from build123d import *

# Parameters (mm, degrees)
SKETCH1_R           = 1.5
BOSS_EXTRUDE1_DEPTH = 1.2
SKETCH2_W           = 29.840930046
SKETCH2_H           = 54.765276652
BOSS_EXTRUDE2_DEPTH = 7
SKETCH3_W           = 33.788082064
SKETCH3_H           = 72.581353001
BOSS_EXTRUDE3_DEPTH = 5.5
SKETCH4_R           = 20
BOSS_EXTRUDE4_DEPTH = 16
SKETCH5_R           = 2.6
BOSS_EXTRUDE5_DEPTH = 6
BOSS_EXTRUDE6_DEPTH = 1.2
FILLET1_R           = 2.5


with BuildPart() as part:
    # Sketch1 → Boss-Extrude1 (new body)
    with BuildSketch(Plane(origin=(0, 0, 0), x_dir=(1, 0, 0), z_dir=(0, 1, 0))):
        with BuildLine():
            Line((2.5, 100), (97.5, 100))
            ThreePointArc((97.5, 100), (99.267766953, 99.267766953), (100, 97.5))
            Line((100, 97.5), (100, 2.5))
            ThreePointArc((100, 2.5), (99.267766953, 0.732233047), (97.5, 0))
            Line((97.5, 0), (2.5, 0))
            ThreePointArc((2.5, 0), (0.732233047, 0.732233047), (0, 2.5))
            Line((0, 2.5), (0, 97.5))
            ThreePointArc((0, 97.5), (0.732233047, 99.267766953), (2.5, 100))
        make_face()
        with Locations((5, 96.3)):
            Circle(SKETCH1_R, mode=Mode.SUBTRACT)
        with Locations((94.6, 95.1)):
            Circle(SKETCH1_R, mode=Mode.SUBTRACT)
        with Locations((5, 3.7)):
            Circle(SKETCH1_R, mode=Mode.SUBTRACT)
        with Locations((94.6, 4.4)):
            Circle(SKETCH1_R, mode=Mode.SUBTRACT)
    extrude(amount=BOSS_EXTRUDE1_DEPTH)

    # Sketch2 → Boss-Extrude2 (add)
    with BuildSketch(Plane.XZ):
        with Locations((36.983095354, -49.21487939)):
            Rectangle(SKETCH2_W, SKETCH2_H)
    extrude(amount=BOSS_EXTRUDE2_DEPTH)

    # Sketch3 → Boss-Extrude3 (add)
    with BuildSketch(Plane.XZ):
        with Locations((79.907693041, -55.955425872)):
            Rectangle(SKETCH3_W, SKETCH3_H)
    extrude(amount=BOSS_EXTRUDE3_DEPTH)

    # Sketch4 → Boss-Extrude4 (add)
    with BuildSketch(Plane(origin=(0, 1.2, 0), x_dir=(1, 0, 0), z_dir=(0, 1, 0))):
        with BuildLine():
            Line((23, -1), (23, 72))
            ThreePointArc((23, 72), (58.049844719, 97.772077914), (72.2, 56.63250183))
            ThreePointArc((72.2, 56.63250183), (69.818614724, 51.754066196), (69, 46.38750305))
            Line((69, 46.38750305), (69, -1))
            Line((69, -1), (23, -1))
        make_face()
        with Locations((50, 72)):
            Circle(SKETCH4_R, mode=Mode.SUBTRACT)
    extrude(amount=BOSS_EXTRUDE4_DEPTH)

    # Sketch5 → Boss-Extrude5 (add)
    with BuildSketch(Plane(origin=(0, 1.2, 0), x_dir=(1, 0, 0), z_dir=(0, 1, 0))):
        with Locations((87.841987056, 95.287894157)):
            Circle(SKETCH5_R)
        with Locations((87.226934535, 5.201319217)):
            Circle(SKETCH5_R)
    extrude(amount=BOSS_EXTRUDE5_DEPTH)

    # Sketch6 → Boss-Extrude6 (add)
    with BuildSketch(Plane(origin=(0, 7.2, 0), x_dir=(1, 0, 0), z_dir=(0, 1, 0))):
        Polygon((80.739794291, 100), (80.739794291, 92.907164266), (79.266881022, 92.907164266), (79.266881022, 48.78574174), (70, 48.78574174), (70, 0), (90.117817522, 0), (90.117817522, 7.917821809), (96.488136969, 7.917821809), (96.488136969, 20.556535591), (100, 20.556535591), (100, 91.38711124), (91.568142489, 91.38711124), (91.568142489, 100), align=None)
    extrude(amount=BOSS_EXTRUDE6_DEPTH)

    # Fillet1
    fillet1_edges = [part.edges().sort_by_distance(p)[0] for p in [
        (90.117817522, 7.8, -7.917821809),
        (96.488136969, 7.8, -7.917821809),
        (91.568142489, 7.8, -91.38711124),
        (91.568142489, 7.8, -100),
        (70, 7.8, -48.78574174),
        (90.117817522, 7.8, 0),
    ]]
    fillet(fillet1_edges, radius=FILLET1_R)


solid = part.part
CAD build for the part. Positions are in the model's coordinates, mm. A direction names the side the tool comes from. Give positions to 0.01 mm unless a question says otherwise; leave off trailing zeros. Write each loop counter-clockwise with the first axis right and the second up, starting at its lowest first coordinate (ties: lowest second). Pieces come first, ordered by that corner, then holes. Notation, with made-up numbers: M -18,37 L -10,37 A27 ccw -10,74 Z; hole C 51.25,41 d9. An arc over 180 degrees is marked long. Put each result on its own line as item: value. Start each with the question number.
(1) Which spindle directions (+Z, -Z, +X, -X, +Y, -Y) get a long thin tool onto all of the face, cutting with end or side? Do faces 5 (the face through (22.063, -3, -50)), 6 (the face through (23, 9, -35)), 7 (the face through (95.775, 7.808, -8.67)). Say none if no direction does.
(2) Band-saw the part on D-D, the plane y = 11.25. Write the cut outline in (x, z), and give its area (3 significant figures).
(3) Band-saw the part on A-A, the plane x = 5. Write the cut outline in (y, z).
(4) Probe L1, parallel to Z at x = 5, y = 0.9; L2, parallel to Z at x = 50, y = 6.5; L3, parallel to Y at x = 89, z = -67.5. List the from-to ranges inside material, lowest first.
(5) Flat gauge pins, fed straight in: pin 1 Ø6 at (x, z) = (15, -31) entering from -Y; pin 2 Ø4 at (x, y) = (72, 8.5) entering from -Z; pin 3 Ø6 at (x, z) = (87.5, -46.5) entering from -Y; pin 4 Ø2.5 at (x, z) = (94.6, -95.1) entering from +Y. Where does each tip first touch, or does it go through?
(6) Mould opens along X. For faces 1 (the face through (89.366, 7.808, -0.713)), 2 (the face through (50, 1.2, -72)), 3 (the face through (0.752, 0.592, -0.713)), 4 (the face through (85, 8.4, -51)) say: +X half, -X half, draft (parallel to the pull), parting line (faces both ways), or undercut.
(7) Band-saw the part on B-B, the plane y = -1.75. Write the cut outline in (x, z), and give its area (3 significant figures).
(8) Band-saw the part on C-C, the plane x = 50. Write the cut outline in (y, z), and give its area (3 significant figures).
Response values:
1. face 5: +Z, -Z, -X, -Y
1. face 6: +Z, -Z, -X, +Y
1. face 7: +Z, +X, +Y
2. outline: M 23,-72 A27 ccw long 72.2,-56.63 A18 cw 69,-46.39 L 69,1 L 23,1 Z; hole C 50,-72 d40
2. area: 3,360 mm2
3. outline: M 0,-100 L 1.2,-100 L 1.2,-97.8 L 0,-97.8 Z; M 0,-94.8 L 1.2,-94.8 L 1.2,-5.2 L 0,-5.2 Z; M 0,-2.2 L 1.2,-2.2 L 1.2,0 L 0,0 Z
4. L1: z = -100 to -97.8, -94.8 to -5.2, -2.2 to 0
4. L2: z = -99 to -92, -52 to 1
4. L3: y = -5.5 to 1.2, 7.2 to 8.4
5. pin 1: stops at y = 0
5. pin 2: stops at z = -90.14
5. pin 3: stops at y = -5.5
5. pin 4: passes through
6. face 1: +X half
6. face 2: undercut
6. face 3: -X half
6. face 4: draft
7. outline: M 22.06,-76.6 L 51.9,-76.6 L 51.9,-21.83 L 22.06,-21.83 Z; M 63.01,-92.25 L 96.8,-92.25 L 96.8,-19.66 L 63.01,-19.66 Z
7. area: 4,090 mm2
8. outline: M -7,-76.6 L 0,-76.6 L 0,-100 L 1.2,-100 L 1.2,-99 L 17.2,-99 L 17.2,-92 L 1.2,-92 L 1.2,-52 L 17.2,-52 L 17.2,1 L 1.2,1 L 1.2,0 L 0,0 L 0,-21.83 L -7,-21.83 Z
8. area: 1,460 mm2
